Input: part model. Units: mm. Frame: model coordinates. Face numbers are marked on the shaded views. A direction names the side the tool comes from. Coordinates: 2 decimals unless noted, no trailing zeros. Write each loop counter-clockwise with the first axis right and the second up, starting at its lowest first coordinate (ties: lowest second). Pieces come first, ordered by that corner, then holes.
from build123d import *

# Parameters (mm, degrees)
F0_R     = 6
F0_R_2   = 2.5
F1_DEPTH = 2
F2_R     = 5.5
F2_R_2   = 3
F3_DEPTH = 0.3


# Not quite as in the source:
# - a pattern or mirror of a feature is missing from the dataset's text; its kind, count and spacing are read off the source's solid


with BuildPart() as f1:
    # F0 (on Front) → F1 (new body, symmetric)
    with BuildSketch(Plane.XZ):
        Circle(F0_R)
        Circle(F0_R_2, mode=Mode.SUBTRACT)
    extrude(amount=F1_DEPTH, both=True)

    # F2 (on face) → F3 (cut)
    with BuildSketch(Plane.XZ.offset(2)):
        Circle(F2_R)
        Circle(F2_R_2, mode=Mode.SUBTRACT)
    f3 = extrude(amount=-F3_DEPTH, mode=Mode.SUBTRACT)

    # F3_copies: F3 across plane
    add(f3.mirror(Plane.ZX), mode=Mode.SUBTRACT)


solid = f1.part
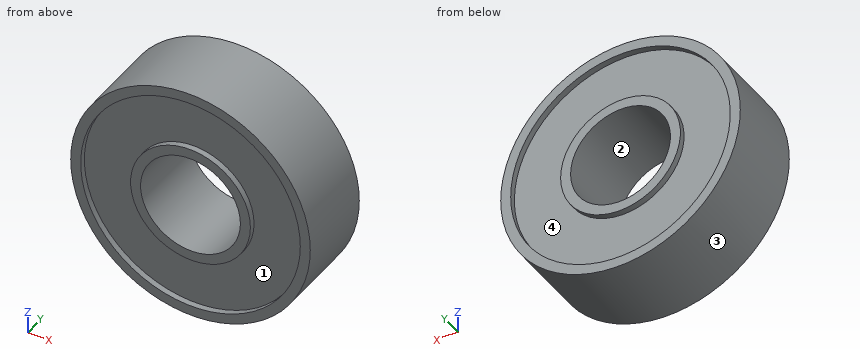
Item 1: Access query for the marked faces 1 and 2. Directions: +Z, -Z, +X, -X, +Y, -Y. A direction counts if a zero-diameter tool reaches every point of the face in a straight line with its end or side. Return the directions, or none.
Item 2: Pin query (flat end, axial travel): pin 1 Ø2 at (y, z) = (1, -2.5) entering from -X; pin 2 Ø1 at (y, z) = (-1, 3) entering from -X; pin 3 Ø1 at (y, z) = (-0.5, 1.5) entering from -X. Return the tip coordinate at first contact, or that it passes through.
Item 3: Section query A-A, the plane z = 0. Return loops of the section in (x, y), then the cut area to 3 significant figures.
Item 4: Section query D-D, the plane x = -2.75. Return loops of the section in (y, z).
Item 5: Section query B-B, the plane x = 0. Return loops of the section in (y, z), then the cut area to 3 significant figures.
Item 6: Section query C-C, the plane y = -0.5. Return loops of the section in (x, z).
Item 7: Material intervals for line 1 (Z direction, x = 0, y = -1.9); line 2 (Z direction, x = 0, y = 1.2); line 3 (X direction, y = 1.75, z = 2.25), sorted ascending.
Item 8: Pull-direction query (X, two-part tool) for the marked faces 3 and 4; classes: released by +X, released by -X, zero draft, split by the parting line, or undercut.
The answers:
1. face 1: -Y
1. face 2: +Y, -Y
2. pin 1: stops at x = -5.81
2. pin 2: stops at x = -5.45
2. pin 3: stops at x = -5.92
3. outline: (-6, -2) - (-5.5, -2) - (-5.5, -1.7) - (-3, -1.7) - (-3, -2) - (-2.5, -2) - (-2.5, 2) - (-3, 2) - (-3, 1.7) - (-5.5, 1.7) - (-5.5, 2) - (-6, 2) - close; (2.5, -2) - (3, -2) - (3, -1.7) - (5.5, -1.7) - (5.5, -2) - (6, -2) - (6, 2) - (5.5, 2) - (5.5, 1.7) - (3, 1.7) - (3, 2) - (2.5, 2) - close
3. area: 25.0 mm2
4. outline: (-2, -5.33) - (2, -5.33) - (2, -4.76) - (1.7, -4.76) - (1.7, -1.2) - (2, -1.2) - (2, 1.2) - (1.7, 1.2) - (1.7, 4.76) - (2, 4.76) - (2, 5.33) - (-2, 5.33) - (-2, 4.76) - (-1.7, 4.76) - (-1.7, 1.2) - (-2, 1.2) - (-2, -1.2) - (-1.7, -1.2) - (-1.7, -4.76) - (-2, -4.76) - close
5. outline: (-2, -6) - (2, -6) - (2, -5.5) - (1.7, -5.5) - (1.7, -3) - (2, -3) - (2, -2.5) - (-2, -2.5) - (-2, -3) - (-1.7, -3) - (-1.7, -5.5) - (-2, -5.5) - close; (-2, 2.5) - (2, 2.5) - (2, 3) - (1.7, 3) - (1.7, 5.5) - (2, 5.5) - (2, 6) - (-2, 6) - (-2, 5.5) - (-1.7, 5.5) - (-1.7, 3) - (-2, 3) - close
5. area: 25.0 mm2
6. outline: circle Ø12 at (0, 0); hole circle Ø5 at (0, 0)
7. line 1: z = -6 to -5.5, -3 to -2.5, 2.5 to 3, 5.5 to 6
7. line 2: z = -6 to -2.5, 2.5 to 6
7. line 3: x = -5.56 to -5.02, -1.98 to -1.09, 1.09 to 1.98, 5.02 to 5.56
8. face 3: split by the parting line
8. face 4: undercut
